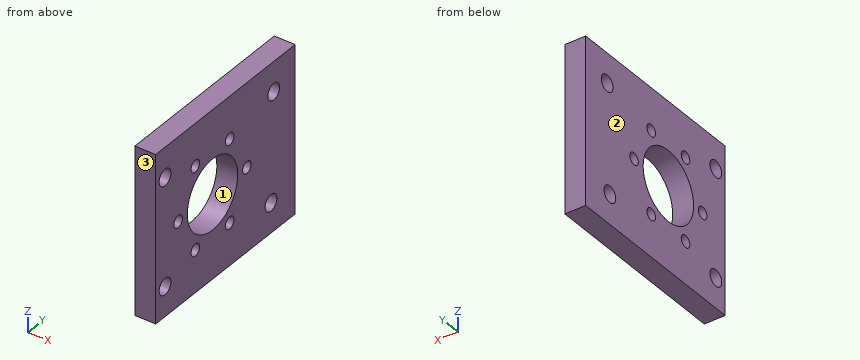
```python
from build123d import *

# Parameters (mm, degrees)
SKETCH1_W           = 56
SKETCH1_H           = 65
BOSS_EXTRUDE1_DEPTH = 7
SKETCH2_R           = 11.75
CUT_EXTRUDE1_DEPTH  = 8
SKETCH3_R           = 2
CUT_EXTRUDE2_DEPTH  = 8
SKETCH4_R           = 2.75
CUT_EXTRUDE3_DEPTH  = 8


with BuildPart() as part:
    # Sketch1 → Boss-Extrude1 (new body)
    with BuildSketch(Plane(origin=(0, 0, 0), x_dir=(0, 0, -1), z_dir=(1, 0, 0))):
        with Locations((28, -32.5)):
            Rectangle(SKETCH1_W, SKETCH1_H)
    extrude(amount=BOSS_EXTRUDE1_DEPTH)

    # Sketch2 → Cut-Extrude1 (cut, through all)
    with BuildSketch(Plane(origin=(7, 0, 0), x_dir=(0, 0, -1), z_dir=(1, 0, 0))):
        with Locations((28, -38.52)):
            Circle(SKETCH2_R)
    extrude(amount=-CUT_EXTRUDE1_DEPTH, mode=Mode.SUBTRACT)

    # Sketch3 → Cut-Extrude2 (cut, through all)
    with BuildSketch(Plane.ZY):
        with Locations((-41.856406461, -30.52)):
            Circle(SKETCH3_R)
        with Locations((-28, -22.52)):
            Circle(SKETCH3_R)
        with Locations((-14.143593539, -30.52)):
            Circle(SKETCH3_R)
        with Locations((-14.143593539, -46.52)):
            Circle(SKETCH3_R)
        with Locations((-28, -54.52)):
            Circle(SKETCH3_R)
        with Locations((-41.856406461, -46.52)):
            Circle(SKETCH3_R)
    extrude(amount=-CUT_EXTRUDE2_DEPTH, mode=Mode.SUBTRACT)

    # Sketch4 → Cut-Extrude3 (cut, through all)
    with BuildSketch(Plane(origin=(7, 0, 0), x_dir=(0, 0, -1), z_dir=(1, 0, 0))):
        with Locations((10, -60.647707201)):
            Circle(SKETCH4_R)
        with Locations((10, -9.998526597)):
            Circle(SKETCH4_R)
        with Locations((46, -11.256698369)):
            Circle(SKETCH4_R)
        with Locations((46, -60.647707201)):
            Circle(SKETCH4_R)
    extrude(amount=-CUT_EXTRUDE3_DEPTH, mode=Mode.SUBTRACT)


solid = part.part
```
Design review of the part built by this model. Coordinates are the model's own, in mm. Face numbers are marked on the shaded views. Round coordinates to 2 decimals unless told otherwise and drop trailing zeros. Write each loop counter-clockwise with the first axis right and the second up, starting at its lowest first coordinate (ties: lowest second). Pieces come first, ordered by that corner, then holes. Notation, with made-up numbers: (63.25, -20.5) -> (87.25, -20.5) arc R18 cw to (87.25, 5.5) -> close; hole circle Ø3 at (-11, 6.5). An arc over 180 degrees is marked (long way). Answer in a Markdown table with one row per item.
Q1. Draft analysis for pull direction Y (two halves, no side actions). For the marked faces 1, 2 and 3, state which applies: +Y half, -Y half, draft (parallel to the pull), parting line (faces both ways), or undercut.
The answers:
| item | result |
|---|---|
| face 1 | undercut |
| face 2 | draft |
| face 3 | -Y half |
Q2. Take a section at B-B, the plane y = -38.52. State the section outline as (x, z) points.
The answers:
| item | result |
|---|---|
| outline | (0, -56) -> (7, -56) -> (7, -39.75) -> (0, -39.75) -> close; (0, -16.25) -> (7, -16.25) -> (7, 0) -> (0, 0) -> close |
Q3. Clearance check with a flat-ended pin moving along its axis: pin 1 Ø3 at (y, z) = (-22.52, -28) entering from -X. State where the tip first meets the part, or that it passes through.
The answers:
| item | result |
|---|---|
| pin 1 | through |
Q4. Take a section at A-A, the plane z = -46. State the section outline as (x, y) points.
The answers:
| item | result |
|---|---|
| outline | (0, -65) -> (7, -65) -> (7, -63.4) -> (0, -63.4) -> close; (0, -57.9) -> (7, -57.9) -> (7, -14.01) -> (0, -14.01) -> close; (0, -8.51) -> (7, -8.51) -> (7, 0) -> (0, 0) -> close |
Q5. To check wall thickness, follow L1, parallel to Y at x = 1.5, z = -46; L2, parallel to Z at x = 2.75, y = -29; L3, parallel to Y at x = 2.25, z = -11.5. State the ranges of each line that lie inside material, in increasing order. Write a range as [from, to].
The answers:
| item | result |
|---|---|
| L1 | [-65, -63.4], [-57.9, -14.01], [-8.51, 0] |
| L2 | [-56, -43.16], [-40.56, -34.89], [-21.11, -15.44], [-12.84, 0] |
| L3 | [-65, -62.95], [-58.34, -12.3], [-7.69, 0] |
Q6. Take a section at C-C, the plane z = -28. State the section outline as (x, y) points, then the cut area to 4 significant figures.
The answers:
| item | result |
|---|---|
| outline | (0, -65) -> (7, -65) -> (7, -56.52) -> (0, -56.52) -> close; (0, -52.52) -> (7, -52.52) -> (7, -50.27) -> (0, -50.27) -> close; (0, -26.77) -> (7, -26.77) -> (7, -24.52) -> (0, -24.52) -> close; (0, -20.52) -> (7, -20.52) -> (7, 0) -> (0, 0) -> close |
| area | 234.5 mm² |
Q7. Take a section at D-D, the plane y = -59. State the section outline as (x, z) points, then the cut area to 3 significant figures.
The answers:
| item | result |
|---|---|
| outline | (0, -56) -> (7, -56) -> (7, -48.2) -> (0, -48.2) -> close; (0, -43.8) -> (7, -43.8) -> (7, -12.2) -> (0, -12.2) -> close; (0, -7.8) -> (7, -7.8) -> (7, 0) -> (0, 0) -> close |
| area | 330 mm² |
